Geometry check sheet. Reference: the model listing, model coordinates, mm. A direction names the side the tool comes from. Coordinates: 2 decimals unless noted, no trailing zeros. Order: outer loops, then holes, each group sorted by start corner. A loop starts at its lowest first (then second) coordinate and runs counter-clockwise, first axis right, second up. Notation, with made-up numbers: M -24.5,9 L -15.5,9 A24 ccw -15.5,34 Z; hole C 74,-12.5 d9. An arc over 180 degrees is marked long. One line per item, written item: value. Start each with the question number.
1) Access from +Z, -Z, +X, -X, +Y, -Y to the whole of each face (thin tool, end or side, straight path). Record for faces 1 (the flat face through (-5, 2, 2)), 2 (the flat face through (-7, 2, 0)), 3 (the flat face through (0.86, 1.76, -5.23)), 4 (the flat face through (-3.4, 0, 0.2)).
2) Sectioned sample at A-A, the plane x = -12. Enter the section's corners in (y, z) (3 decimals).
3) Draft check along Z on faces 5 (the flat face through (-6, 2, 3.5)), 6 (the flat face through (-15, 1.7, 0.9)), 7 (the flat face through (-0.47, 2.5, -15.15)), 8 (the flat face through (-1.32, 1.73, -7.49)). Enter one of: pulls with the +Z half, pulls with the -Z half, needs draft (parallel to the pull), parting line crosses it, or undercut.
4) Thickness scan on L1, parallel to Z at x = -8.5, y = 0.4; L2, parallel to Z at x = -12.5, y = 2.05; L3, parallel to X at y = 2.3, z = -11. Record the ranges inside material, lowest first. Write a range as from..to.
5) Sectioned sample at B-B, the plane y = 2.05. Enter the section's corners in (x, z), then the cut area to 3 significant figures.
6) Go/stop test with a flat-tipped pin: P1, Ø1.5, axis at x = -4.5, y = 3, coming from the -Z side. Record where the tip stops, or that it passes through.
7) Sectioned sample at D-D, the plane x = 2.75. Enter the section's corners in (y, z), then the cut area to 3 significant figures.
8) Sectioned sample at C-C, the plane z = -4. Enter the section's corners in (x, y).
```python
from build123d import *

# Parameters (mm, degrees)
BOSS_EXTRUDE1_DEPTH = 3.5
CUT_EXTRUDE1_DEPTH  = 10
CUT_EXTRUDE3_DEPTH  = 10


with BuildPart() as part:
    # Sketch2 → Boss-Extrude1 (new body)
    with BuildSketch(Plane(origin=(0, 0, 0), x_dir=(1, 0, 0), z_dir=(0, 1, 0))):
        Polygon((0, 0), (-15, 0), (-15, -3.5), (4.171137574, -3.5), (0.842104471, 15.379884917), (-2.604722665, 14.772116295), align=None)
    extrude(amount=BOSS_EXTRUDE1_DEPTH)

    # Sketch3 → Cut-Extrude1 (cut)
    with BuildSketch(Plane.ZY.offset(15)):
        with BuildLine():
            ThreePointArc((2.425, 1.75), (2.227297077, 2.227297077), (1.75, 2.425))
            Line((1.75, 2.425), (1.75, 1.075))
            ThreePointArc((1.75, 1.075), (2.227297077, 1.272702923), (2.425, 1.75))
        make_face()
        with BuildLine():
            Line((1.75, 1.075), (1.75, 2.425))
            ThreePointArc((1.75, 2.425), (1.272702923, 2.227297077), (1.075, 1.75))
            ThreePointArc((1.075, 1.75), (1.272702923, 1.272702923), (1.75, 1.075))
        make_face()
    extrude(amount=-CUT_EXTRUDE1_DEPTH, mode=Mode.SUBTRACT)

    # Sketch4 → Cut-Extrude3 (cut)
    with BuildSketch(Plane(origin=(-2.604722665, 0, -14.772116295), x_dir=(-0.984807753, 0, 0.173648178), z_dir=(-0.173648178, 0, -0.984807753))):
        with BuildLine():
            ThreePointArc((-1.075, 1.75), (-1.272702923, 2.227297077), (-1.75, 2.425))
            Line((-1.75, 2.425), (-1.75, 1.075))
            ThreePointArc((-1.75, 1.075), (-1.272702923, 1.272702923), (-1.075, 1.75))
        make_face()
        with BuildLine():
            Line((-1.75, 1.075), (-1.75, 2.425))
            ThreePointArc((-1.75, 2.425), (-2.227297077, 2.227297077), (-2.425, 1.75))
            ThreePointArc((-2.425, 1.75), (-2.227297077, 1.272702923), (-1.75, 1.075))
        make_face()
    extrude(amount=-CUT_EXTRUDE3_DEPTH, mode=Mode.SUBTRACT)


solid = part.part
```
Final values:
1. face 1: -X
1. face 2: -X, +Y, -Y
1. face 3: none
1. face 4: +Z, -Z, +X, -X, -Y
2. outline: M 0,0 L 3.5,0 L 3.5,3.5 L 0,3.5 Z; hole C 1.75,1.75 d1.35
3. face 5: pulls with the +Z half
3. face 6: needs draft
3. face 7: pulls with the -Z half
3. face 8: undercut
4. L1: z = 0..3.5
4. L2: z = 0..1.15, 2.35..3.5
4. L3: x = -1.94..-0.56, 0.23..1.61
5. outline: M -15,0 L 0,0 L -2.6,-14.77 L -1.48,-14.97 L 0.26,-5.12 L 1.45,-5.33 L -0.29,-15.18 L 0.84,-15.38 L 4.17,3.5 L -15,3.5 L -15,2.35 L -5,2.35 L -5,1.15 L -15,1.15 Z
5. area: 95.4 mm^2
6. P1: stops at z = 0
7. outline: M 0,-4.56 L 3.5,-4.56 L 3.5,3.5 L 0,3.5 Z
7. area: 28.2 mm^2
8. outline: M -0.71,0 L 2.85,0 L 2.85,3.5 L -0.71,3.5 Z
